```python
from build123d import *

# Parameters (mm, degrees)
F1_DEPTH = 4.7625
F2_ANGLE = 270


with BuildPart() as f1:
    # F0 (on Front) → F1 (new body)
    with BuildSketch(Plane.XZ):
        with BuildLine():
            Line((-230.3694504243, 0), (-611.3694504243, 0))
            Line((-611.3694504243, 0), (-611.3694504243, -76.2))
            ThreePointArc((-611.3694504243, -76.2), (-437.216196434, -280.1613571834), (-193.5208703627, -392.1532280958))
            Line((-193.5208703627, -392.1532280958), (-193.5208703627, -244.9399656624))
            Line((-193.5208703627, -244.9399656624), (-168.1208703627, -244.9399656624))
            Line((-168.1208703627, -244.9399656624), (-166.920896507, -397.3352413856))
            ThreePointArc((-166.920896507, -397.3352413856), (-114.1339631712, -404.1296791803), (-60.96, -406.4))
            Line((-60.96, -406.4), (0, -406.4))
            Line((0, -406.4), (0, -342.9))
            Line((0, -342.9), (-127, -342.9))
            Line((-127, -342.9), (-127, -279.4))
            Line((-127, -279.4), (0, -279.4))
            Line((0, -279.4), (0, -228.6))
            Line((0, -228.6), (-127, -228.6))
            Line((-127, -228.6), (-127, -165.1))
            Line((-127, -165.1), (0, -165.1))
            Line((0, -165.1), (0, -114.3))
            Line((0, -114.3), (-127, -114.3))
            Line((-127, -114.3), (-127, -50.8))
            Line((-127, -50.8), (0, -50.8))
            Line((0, -50.8), (0, 0))
            Line((0, 0), (-208.5918039083, 0))
            Line((-208.5918039083, 0), (-208.5918039083, -152.4))
            Line((-208.5918039083, -152.4), (-230.3694504243, -152.4))
            Line((-230.3694504243, -152.4), (-230.3694504243, 0))
        make_face()
    extrude(amount=F1_DEPTH)


with BuildPart() as f1_1:
    # F2: moved
    add(f1.part.rotate(Axis((0, 0, -139.7), (0, 0, 1)), F2_ANGLE))


solid = f1_1.part
```
Input: part model. Units: mm. Frame: model coordinates. Give positions to 0.01 mm unless a question says otherwise; leave off trailing zeros. Order: outer loops, then holes, each group sorted by start corner. A loop starts at its lowest first (then second) coordinate and runs counter-clockwise, first axis right, second up. Notation, with made-up numbers: (46, 62) - (72, 62) arc R22 cw to (72, 79) - close; hole circle Ø1 at (70.25, 77.25). An arc over 180 degrees is marked (long way). Use a Markdown table: item, result.
(1) Pin query (flat end, axial travel): pin 1 (1.5 mm diameter, centred on x = -2.5, y = 515.5, fed in from -Z); pin 2 (1.4 mm diameter, centred on x = -3, y = 77, fed in from -Z). Return the tip coordinate at first contact, or that it passes through.
Computed values:
| item | result |
|---|---|
| pin 1 | stops at z = -210.64 |
| pin 2 | stops at z = -406.21 |
(2) Section query B-B (y = 67.5). Output: boundary loops of the cut face in (x, z).
Computed values:
| item | result |
|---|---|
| outline | (-4.76, -406.37) - (0, -406.37) - (0, -342.9) - (-4.76, -342.9) - close; (-4.76, -279.4) - (0, -279.4) - (0, -228.6) - (-4.76, -228.6) - close; (-4.76, -165.1) - (0, -165.1) - (0, -114.3) - (-4.76, -114.3) - close; (-4.76, -50.8) - (0, -50.8) - (0, 0) - (-4.76, 0) - close |
(3) Line query: line 1 (Y direction, x = -1.4, z = -39); line 2 (Y direction, x = -0.65, z = -90); line 3 (Z direction, x = -4.6, y = 173). Output: solid intervals per line, ascending. Write a range as from..to.
Computed values:
| item | result |
|---|---|
| line 1 | y = 0..208.59, 230.37..611.37 |
| line 2 | y = 127..208.59, 230.37..603.78 |
| line 3 | z = -244.94..0 |
(4) Section query D-D (z = -298.5). Output: boundary loops of the cut face in (x, y).
Computed values:
| item | result |
|---|---|
| outline | (-4.76, 127) - (0, 127) - (0, 167.7) - (-4.76, 167.7) - close; (-4.76, 193.52) - (0, 193.52) - (0, 411.65) - (-4.76, 411.65) - close |
(5) Section query C-C (x = -3.35). Output: boundary loops of the cut face in (y, z), then the cut area to 3 significant figures.
Computed values:
| item | result |
|---|---|
| outline | (0, -406.4) - (60.96, -406.4) arc R623.84 ccw to (166.92, -397.34) - (168.12, -244.94) - (193.52, -244.94) - (193.52, -392.15) arc R623.84 ccw to (611.37, -76.2) - (611.37, 0) - (230.37, 0) - (230.37, -152.4) - (208.59, -152.4) - (208.59, 0) - (0, 0) - (0, -50.8) - (127, -50.8) - (127, -114.3) - (0, -114.3) - (0, -165.1) - (127, -165.1) - (127, -228.6) - (0, -228.6) - (0, -279.4) - (127, -279.4) - (127, -342.9) - (0, -342.9) - close |
| area | 165,000 mm2 |
(6) Section query A-A (z = -24). Output: boundary loops of the cut face in (x, y).
Computed values:
| item | result |
|---|---|
| outline | (-4.76, 0) - (0, 0) - (0, 208.59) - (-4.76, 208.59) - close; (-4.76, 230.37) - (0, 230.37) - (0, 611.37) - (-4.76, 611.37) - close |
